Source: CAD feature listing. Evaluate the final solid. Frame: model axes, mm. Face numbers are marked on the shaded views. A direction names the side the tool comes from. Coordinates: 2 decimals unless noted, no trailing zeros. Order: outer loops, then holes, each group sorted by start corner. A loop starts at its lowest first (then second) coordinate and runs counter-clockwise, first axis right, second up. Notation, with made-up numbers: (63, -11) -> (94, -11) arc R33 cw to (94, 28) -> close; hole circle Ø5 at (39, -22.5). An arc over 180 degrees is marked (long way). Write item = value, one per line. Start each with the question number.
Item 1: Ray query, line 1 along Y through (x, z) = (2, 11); line 2 along Z through (x, y) = (27, 11); line 3 along X through (y, z) = (9, 35.5). Return the intervals inside material, ascending. Write a range as [from, to].
Item 2: Section query D-D (z = 32.7). Output: boundary loops of the cut face in (x, y).
Item 3: Set-up query: the marked faces 4, 5 and 6. Return all of +Z, -Z, +X, -X, +Y, -Y with unobstructed straight access to the full face (end or side cutting, diameter ignored); none if empty.
Item 4: Section query A-A (y = 15.5). Output: boundary loops of the cut face in (x, z), then the cut area to 3 significant figures.
Item 5: Contact query for flat-ended pins moving along their axis: pin 1 (4.5 mm diameter, centred on x = 15.2, y = -8.75, fed in from +Z); pin 2 (2.5 mm diameter, centred on y = -10.5, z = -11, fed in from +X); pin 3 (4 mm diameter, centred on y = -8.75, z = 32.7, fed in from +X); pin 4 (16.5 mm diameter, centred on x = 15.5, y = -1, fed in from -Z). Output: stop coordinate, or through.
Item 6: Section query C-C (x = 9). Output: boundary loops of the cut face in (y, z), then the cut area to 3 significant figures.
Item 7: Mould query, pull axis X, two halves, no side actions, for the marked faces 1, 2 and 3. Classes: released by +X, released by -X, zero draft, split by the parting line, or undercut.
Item 8: Section query B-B (z = 0). Output: boundary loops of the cut face in (x, y), then the cut area to 3 significant figures.
Autodesk Fusion 360 part; units mm, degrees
sketch "스케치1" plane through (0, 0, 0) normal (1, 0, 0) x (0, 1, 0)
  line L0 (10.5, 11) -> (-10.5, 11)
  line L1 (-10.5, 11) -> (-10.5, -11)
  line L2 (-10.5, -11) -> (10.5, -11)
  line L3 (10.5, -11) -> (10.5, 11)
  line L4 (10.5, 11) -> (-10.5, -11) construction
  line L5 (-10.5, 11) -> (10.5, -11) construction
  circle A0 centre (10.5, 11) radius 1.5
  circle A1 centre (-10.5, 11) radius 1.5
  circle A2 centre (10.5, -11) radius 1.5
  circle A3 centre (-10.5, -11) radius 1.5
  line L6 (10.5, 0) -> (1.5, 0)
  circle A4 centre (1.5, 0) radius 6
  line L7 (10.5, 0) -> (18.5, 0)
  line L8 (1.5, 0) -> (-16, 0)
  line L9 (18.5, 0) -> (18.5, 17.5)
  line L10 (-16, 0) -> (-16, -17.5)
  line L11 (-16, -17.5) -> (18.5, -17.5)
  line L12 (18.5, -17.5) -> (18.5, 17.5)
  line L13 (18.5, 17.5) -> (-16, 17.5)
  line L14 (-16, 17.5) -> (-16, -17.5)
  line L15 (-16, 17.5) -> (18.5, 17.5)
  line L16 (18.5, 17.5) -> (18.5, 47.9)
  line L17 (18.5, 47.9) -> (-16, 47.9)
  line L18 (-16, 47.9) -> (-16, 17.5)
  dimension "d1" = 21
  dimension "d2" = 22
  dimension "d3" = 3
  dimension "d4" = 3
  dimension "d5" = 3
  dimension "d6" = 3
  dimension "d8" = 9
  dimension "d9" = 12
  dimension "d10" = 8
  dimension "d11" = 17.5
  dimension "d12" = 17.5
  dimension "d13" = 17.5
  dimension "d16" = 30.4
extrude "돌출1" add sketch "스케치1" along normal blind 3 contours L0 L1 L3 A0 A1 L7 L8 L9 L12 L13 L14 L15 | L0 L1 L3 A0 A1 L6 A4 L8 | L1 L2 L3 A2 A3 L6 A4 L8 | L1 L2 L3 A2 A3 L7 L8 L10 L11 L12 L14 | L13 L15 L16 L17 L18
extrude "돌출2" add sketch "스케치1" along normal blind 30.4 contours L13 L15 L16 L17 L18
sketch "스케치5" plane through (0, 18.5, 0) normal (0, 1, 0) x (-1, 0, 0)
  line L0 (-3, 17.5) -> (-3, -17.5)
  line L1 (-3, -17.5) -> (0, -17.5)
  line L2 (0, -17.5) -> (0, 47.9)
  line L3 (0, 47.9) -> (-30.4, 47.9)
  line L4 (-30.4, 47.9) -> (-30.4, 17.5)
  line L5 (-30.4, 17.5) -> (-3, 17.5)
  line L6 (-30.4, 47.9) -> (0, 47.9)
  line L7 (0, 47.9) -> (0, 17.5)
  line L8 (0, 17.5) -> (-30.4, 17.5)
  line L9 (-30.4, 17.5) -> (-30.4, 47.9)
  line L10 (-5, 42.9) -> (-25.4, 42.9)
  line L11 (-25.4, 42.9) -> (-25.4, 22.5)
  line L12 (-25.4, 22.5) -> (-5, 22.5)
  line L13 (-5, 22.5) -> (-5, 42.9)
  line L14 (-5, 42.9) -> (-25.4, 22.5) construction
  line L15 (-25.4, 42.9) -> (-5, 22.5) construction
  point P0 (-15.2, 32.7)
  dimension "d37" = 20.4
  dimension "d38" = 20.4
extrude "돌출7" cut sketch "스케치5" against normal blind 100 contours L10 L11 L12 L13
sketch "스케치6" plane through (0, 0, 47.9) normal (0, 0, 1) x (-1, 0, 0)
  line L0 (0, -18.5) -> (0, 16)
  line L1 (0, 16) -> (-30.4, 16)
  line L2 (-30.4, 16) -> (-30.4, -18.5)
  line L3 (-30.4, -18.5) -> (0, -18.5)
  line L4 (-15.2, 16) -> (-15.2, 8.75)
  circle A0 centre (-15.2, 8.75) radius 2.6
  line L5 (-15.2, -18.5) -> (-15.2, -11.25)
  circle A1 centre (-15.2, -11.25) radius 2.6
  dimension "d41" = 7.25
  dimension "d42" = 5.2
  dimension "d43" = 7.25
  dimension "d44" = 5.2
extrude "돌출8" cut sketch "스케치6" against normal blind 5 contours A0 | A1
sketch "스케치7" plane through (30.4, 0, 0) normal (1, 0, 0) x (0, 1, 0)
  line L0 (-16, 47.9) -> (-16, 17.5)
  line L1 (-16, 17.5) -> (18.5, 17.5)
  line L2 (18.5, 17.5) -> (18.5, 47.9)
  line L3 (18.5, 47.9) -> (-16, 47.9)
  line L4 (-16, 32.7) -> (-8.75, 32.7)
  circle A0 centre (-8.75, 32.7) radius 2.6
  line L5 (18.5, 32.7) -> (11.25, 32.7)
  circle A1 centre (11.25, 32.7) radius 2.6
  dimension "d47" = 7.25
  dimension "d48" = 5.2
  dimension "d49" = 7.25
  dimension "d50" = 5.2
extrude "돌출9" cut sketch "스케치7" against normal blind 5 contours A0 | A1
extrude "돌출6" [suppressed]
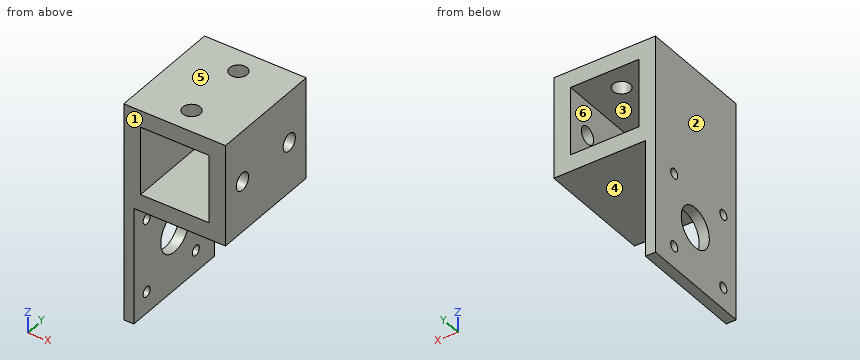
Computed:
q1.line_1 = [-16, -12], [-9, 9], [12, 18.5]
q1.line_2 = [17.5, 30.11], [35.29, 47.9]
q1.line_3 = [0, 5], [25.4, 30.4]
q2.outline = (0, -16) -> (5, -16) -> (5, 18.5) -> (0, 18.5) -> close; (25.4, -16) -> (30.4, -16) -> (30.4, -11.35) -> (25.4, -11.35) -> close; (25.4, -6.15) -> (30.4, -6.15) -> (30.4, 8.65) -> (25.4, 8.65) -> close; (25.4, 13.85) -> (30.4, 13.85) -> (30.4, 18.5) -> (25.4, 18.5) -> close
q3.face_4 = -Z, +X, +Y, -Y
q3.face_5 = +Z, +X, -X, +Y, -Y
q3.face_6 = +Y, -Y
q4.outline = (0, -17.5) -> (3, -17.5) -> (3, 17.5) -> (30.4, 17.5) -> (30.4, 47.9) -> (0, 47.9) -> close; hole (5, 22.5) -> (25.4, 22.5) -> (25.4, 42.9) -> (5, 42.9) -> close
q4.area = 613 mm^2
q5.pin_1 = 22.5
q5.pin_2 = through
q5.pin_3 = 5
q5.pin_4 = 17.5
q6.outline = (-16, 17.5) -> (18.5, 17.5) -> (18.5, 22.5) -> (-16, 22.5) -> close; (-16, 42.9) -> (18.5, 42.9) -> (18.5, 47.9) -> (-16, 47.9) -> close
q6.area = 345 mm^2
q7.face_1 = zero draft
q7.face_2 = released by -X
q7.face_3 = undercut
q8.outline = (0, -16) -> (3, -16) -> (3, -4.5) -> (0, -4.5) -> close; (0, 7.5) -> (3, 7.5) -> (3, 18.5) -> (0, 18.5) -> close
q8.area = 67.5 mm^2
